Build history of the part. All positions in model axes, mm. Face numbers are marked on the shaded views. A direction names the side the tool comes from. Coordinates: 2 decimals unless noted, no trailing zeros. Loops run counter-clockwise (first coordinate to the right, second up) from the corner with the lowest first, then second, coordinate; pieces in that order, holes last.
(1) Two-plate mould, pull along X, no slides. Class the marked faces 4, 5, 6 and 7: pulls with the +X half, pulls with the -X half, needs draft (parallel to the pull), parting line crosses it, or undercut.
(2) Slice it at D-D (z = -7). Give the cut face in (x, y), and give its area (3 significant figures).
(3) Slice it at B-B (x = -18). Give the cut face in (y, z), and give its area (3 significant figures).
(4) Wall check: L1, parallel to X at y = 6.5, z = 0; L2, parallel to X at y = 18.25, z = 0; L3, parallel to X at y = 15.25, z = -3.5. Give the ranges that are in metal, low to high.
(5) Slice it at A-A (z = 0). Give the cut face in (x, y), and give its area (3 significant figures).
(6) Tool access for the marked faces 1, 2 and 3: list every direction of +Z, -Z, +X, -X, +Y, -Y with a clear straight run to the whole face (end or side of a thin tool).
(7) Slice it at C-C (y = 3.5). Give the cut face in (x, z).
(8) Flat gauge pins, fed straight in: P1, Ø9.5, axis at y = 8.5, z = -3.5, coming from the +X side; P2, Ø5, axis at y = 12, z = 29.5, coming from the -X side; P3, Ø9, axis at y = 9.5, z = -3, coming from the -X side; P4, Ø10, axis at y = 18, z = 1.5, coming from the -X side. Where does each tip first touch, or does it go through?
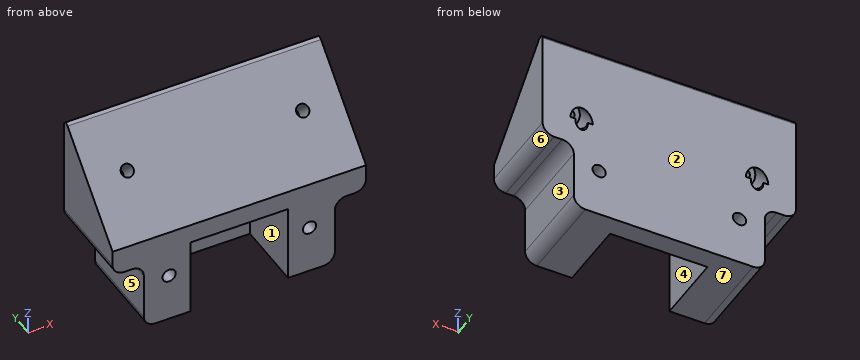
from build123d import *

# Parameters (mm, degrees)
SKETCH_1_W               = 65
SKETCH_1_H               = 25
EXTRUDE_1_DEPTH          = 23
EXTRUDE_2_DEPTH          = 65
SKETCH_3_W               = 25
SKETCH_3_H               = 20
CUT_EXTRUDE_1_DEPTH      = 18
CUT_EXTRUDE_2_DEPTH      = 53.605845683
CUT_EXTRUDE_2_DEPTH_BACK = 53.605845683
SKETCH_4_R               = 1.6
CUT_EXTRUDE_START        = -7
SKETCH_5_R               = 2.9
CUT_EXTRUDE_3_DEPTH      = 9
CUT_EXTRUDE_4_DEPTH      = 54.343228249
CUT_EXTRUDE_4_DEPTH_BACK = 54.343228249
SKETCH_6_R               = 1.7
FILLET_1_R               = 1
SKETCH_7_W               = 8
SKETCH_7_H               = 18
CUT_EXTRUDE_5_DEPTH      = 40
FILLET_2_R               = 3


with BuildPart() as part:
    # 草图1 → 凸台-拉伸1 (new body)
    with BuildSketch(Plane(origin=(0, 0, 0), x_dir=(1, 0, 0), z_dir=(0, 1, 0))):
        Rectangle(SKETCH_1_W, SKETCH_1_H)
    extrude(amount=EXTRUDE_1_DEPTH)

    # 草图2 → 凸台-拉伸2 (add)
    with BuildSketch(Plane(origin=(32.5, 0, 0), x_dir=(0, 0, -1), z_dir=(1, 0, 0))):
        Polygon((-12.5, 0), (-35.5, 23), (-12.5, 23), align=None)
    extrude(amount=-EXTRUDE_2_DEPTH)

    # 草图3 → 切除-拉伸1 (cut)
    with BuildSketch(Plane.XZ):
        with Locations((0, -2.5)):
            Rectangle(SKETCH_3_W, SKETCH_3_H)
    extrude(amount=-CUT_EXTRUDE_1_DEPTH, mode=Mode.SUBTRACT)

    # 草图4 → 切除-拉伸2 (cut, two sides: drawn at the far end of the back side and taken through both)
    with BuildSketch(Plane(origin=(0, -6.25, 6.25), x_dir=(1, 0, 0), z_dir=(0, -0.7071067811865489, 0.7071067811865462)).offset(-CUT_EXTRUDE_2_DEPTH_BACK)):
        with Locations(Location((-22.5, 25.102290732, 0), (0, 0, 270))):
            Circle(SKETCH_4_R)
        with Locations(Location((22.5, 25.102290732, 0), (0, 0, 270))):
            Circle(SKETCH_4_R)
    extrude(amount=CUT_EXTRUDE_2_DEPTH + CUT_EXTRUDE_2_DEPTH_BACK, mode=Mode.SUBTRACT)

    # 草图5 → 切除-拉伸3 (cut)
    with BuildSketch(Plane(origin=(0, -6.25, 6.25), x_dir=(1, 0, 0), z_dir=(0, -0.7071067811865489, 0.7071067811865462)).offset(CUT_EXTRUDE_START)):
        with Locations(Location((-22.5, 25.102290732, 0), (0, 0, 270))):
            Circle(SKETCH_5_R)
        with Locations(Location((22.5, 25.102290732, 0), (0, 0, 174.787670359))):
            Circle(SKETCH_5_R)
    extrude(amount=-CUT_EXTRUDE_3_DEPTH, mode=Mode.SUBTRACT)

    # 草图6 → 切除-拉伸4 (cut, two sides: drawn at the far end of the back side and taken through both)
    with BuildSketch(Plane.XZ.offset(-CUT_EXTRUDE_4_DEPTH_BACK)):
        with Locations(Location((-18, 0, 0), (0, 0, 270))):
            Circle(SKETCH_6_R)
        with Locations(Location((18, 0, 0), (0, 0, 270))):
            Circle(SKETCH_6_R)
    extrude(amount=CUT_EXTRUDE_4_DEPTH + CUT_EXTRUDE_4_DEPTH_BACK, mode=Mode.SUBTRACT)

    # 圆角1
    fillet_1_edges = [part.edges().sort_by_distance(p)[0] for p in [
        (0, 23, 35.5),
    ]]
    fillet(fillet_1_edges, radius=FILLET_1_R)

    # 草图7 → 切除-拉伸5 (cut)
    with BuildSketch(Plane(origin=(0, 23, 0), x_dir=(1, 0, 0), z_dir=(0, 1, 0))):
        with Locations((-28.5, 3.5)):
            Rectangle(SKETCH_7_W, SKETCH_7_H)
        with Locations((28.5, 3.5)):
            Rectangle(SKETCH_7_W, SKETCH_7_H)
    extrude(amount=-CUT_EXTRUDE_5_DEPTH, mode=Mode.SUBTRACT)

    # 圆角2
    fillet_2_edges = [part.edges().sort_by_distance(p)[0] for p in [
        (-32.5, 11.5, 5.5),
        (-24.5, 11.5, -12.5),
        (-24.5, 11.5, 5.5),
        (24.5, 11.5, -12.5),
        (32.5, 11.5, 5.5),
        (24.5, 11.5, 5.5),
    ]]
    fillet(fillet_2_edges, radius=FILLET_2_R)


solid = part.part
Response values:
1. face 4: undercut
1. face 5: pulls with the -X half
1. face 6: pulls with the +X half
1. face 7: needs draft
2. outline: (-24.5, 0) - (-12.5, 0) - (-12.5, 18) - (12.5, 18) - (12.5, 0) - (24.5, 0) - (24.5, 23) - (-24.5, 23) - close
2. area: 677 mm2
3. outline: (0, -12.5) - (23, -12.5) - (23, -1.7) - (0, -1.7) - close; (0, 1.7) - (23, 1.7) - (23, 33.09) arc R1 ccw to (21.29, 33.79) - (0, 12.5) - close
3. area: 760 mm2
4. L1: x = -24.5 to -19.7, -16.3 to -12.5, 12.5 to 16.3, 19.7 to 24.5
4. L2: x = -24.5 to -19.7, -16.3 to 16.3, 19.7 to 24.5
4. L3: x = -24.5 to -12.5, 12.5 to 24.5
5. outline: (-24.5, 0) - (-19.7, 0) - (-19.7, 23) - (-24.5, 23) - close; (-16.3, 0) - (-12.5, 0) - (-12.5, 18) - (12.5, 18) - (12.5, 0) - (16.3, 0) - (16.3, 23) - (-16.3, 23) - close; (19.7, 0) - (24.5, 0) - (24.5, 23) - (19.7, 23) - close
5. area: 521 mm2
6. face 1: -Z, -Y
6. face 2: +Z, -Z, +X, -X, +Y
6. face 3: -Z, +X, +Y, -Y
7. outline: (-32.5, 8.5) arc R3 ccw to (-29.5, 5.5) - (-27.5, 5.5) arc R3 cw to (-24.5, 2.5) - (-24.5, -9.5) arc R3 ccw to (-21.5, -12.5) - (-12.5, -12.5) - (-12.5, 7.5) - (12.5, 7.5) - (12.5, -12.5) - (21.5, -12.5) arc R3 ccw to (24.5, -9.5) - (24.5, 2.5) arc R3 cw to (27.5, 5.5) - (29.5, 5.5) arc R3 ccw to (32.5, 8.5) - (32.5, 16) - (-32.5, 16) - close; hole circle Ø3.4 at (-18, 0); hole circle Ø3.4 at (18, 0)
8. P1: stops at x = 24.5
8. P2: passes through
8. P3: stops at x = -24.5
8. P4: stops at x = -31.74
